Autodesk Inventor part; units mm, degrees
ref_plane "YZ Plane" through (0, 0, 0) normal (1, 0, 0) x (0, 1, 0)
ref_plane "XZ Plane" through (0, 0, 0) normal (0, 1, 0) x (-1, 0, 0)
ref_plane "XY Plane" through (0, 0, 0) normal (0, 0, 1) x (1, 0, 0)
sketch "Sketch1" plane through (0, 0, 0) normal (0, 1, 0) x (-1, 0, 0)
  point P0 (0, 0)
sketch "Sketch2" plane through (0, 0, 0) normal (0, 1, 0) x (-1, 0, 0)
  line L0 (-63.5, 112) -> (63.5, 112)
  line L1 (63.5, 112) -> (63.5, -112)
  line L2 (63.5, -112) -> (-63.5, -112)
  line L3 (-63.5, -112) -> (-63.5, 112)
  line L4 (-63.5, 112) -> (63.5, -112) construction
  line L5 (63.5, 112) -> (-63.5, -112) construction
  point P0 (0, 0)
  dimension "d0" = 127
  dimension "d1" = 224
extrude "Extrusion1" add sketch "Sketch2" along normal blind 76.2
sketch "Sketch3" plane through (0, 76.2, 0) normal (0, 1, 0) x (1, 0, 0)
  line L0 (59.69, 107.95) -> (-59.69, 107.95)
  line L1 (-59.69, 107.95) -> (-59.69, -107.95)
  line L2 (-59.69, -107.95) -> (59.69, -107.95)
  line L3 (59.69, -107.95) -> (59.69, 107.95)
  line L4 (59.69, 107.95) -> (-59.69, -107.95) construction
  line L5 (-59.69, 107.95) -> (59.69, -107.95) construction
  point P0 (0, 0)
  dimension "d4" = 119.38
  dimension "d5" = 215.9
extrude "Extrusion2" cut sketch "Sketch3" against normal blind 73.66
sketch "Sketch4" plane through (-59.69, 76.2, -107.95) normal (0, 0, 1) x (1, 0, 0)
  line L0 (119.38, 0) -> (119.38, -73.66)
  line L1 (119.38, 0) -> (0, 0)
  line L2 (0, 0) -> (0, -5.08)
  line L3 (0, -5.08) -> (119.38, -5.08)
  line L4 (119.38, -5.08) -> (119.38, 0)
  point P0 (59.69, -76.2)
  dimension "d8" = 5.08
  dimension "d11" = 119.38
extrude "Extrusion3" add sketch "Sketch4" along normal blind 38.1
sketch "Sketch5" plane through (59.69, 76.2, 107.95) normal (0, 0, -1) x (-1, 0, 0)
  line L0 (0, 0) -> (119.38, 0)
  line L1 (119.38, 0) -> (119.38, -5.08)
  line L2 (119.38, -5.08) -> (0, -5.08)
  line L3 (0, -5.08) -> (0, 0)
  point P0 (59.69, -76.2)
  dimension "d12" = 5.08
extrude "Extrusion4" add sketch "Sketch5" along normal blind 38.1
sketch "Sketch7" plane through (63.5, 0, 112) normal (1, 0, 0) x (0, 0, -1)
  line L0 (224, 0) -> (0, 0)
  line L1 (224, 0) -> (224, 76.2)
  line L2 (0, 76.2) -> (224, 76.2)
  line L3 (0, 0) -> (0, 76.2)
  point P0 (112, 0)
extrude "Extrusion5" cut sketch "Sketch7" against normal blind 5.08
sketch "Sketch8" plane through (-59.69, 76.2, -69.85) normal (0, 0, 1) x (1, 0, 0)
  line L0 (0, -5.08) -> (118.11, -5.08)
  line L1 (118.11, 0) -> (0, 0)
  line L2 (118.11, -5.08) -> (92.71, -5.08)
  line L3 (92.71, -5.08) -> (92.71, 0)
  line L4 (92.71, 0) -> (118.11, 0)
  line L5 (118.11, 0) -> (118.11, -5.08)
  point P0 (59.69, -76.2)
  dimension "d17" = 25.4
extrude "Extrusion6" add sketch "Sketch8" along normal blind 139.7
sketch "Sketch9" plane through (58.42, 0, 112) normal (1, 0, 0) x (0, 0, -1)
  line L0 (219.95, 2.54) -> (219.95, 71.12)
  line L1 (219.95, 2.54) -> (4.05, 2.54)
  line L2 (4.05, 2.54) -> (4.05, 0)
  line L3 (4.05, 0) -> (219.95, 0)
  line L4 (219.95, 0) -> (219.95, 2.54)
  point P0 (112, 0)
extrude "Extrusion7" cut sketch "Sketch9" against normal blind 71.12
fillet "Fillet1" radius 3.175 1 edges at (58.42, 71.12, 0)
fillet "Fillet2" radius 3.175 1 edges at (-13.335, 71.12, -69.85)
fillet "Fillet3" radius 3.175 1 edges at (-13.335, 71.12, 69.85)
sketch "Sketch10" plane through (-63.5, 0, -112) normal (0, 0, -1) x (-1, 0, 0)
  circle A0 centre (-102.87, 19.05) radius 4
  point P0 (-63.5, 0)
  dimension "d27" = 8
hole "Hole1" at (39.37, 19.05, -112) direction (0, 0, 1) diameter 8 end through all
fillet "Fillet4" radius 3.175 1 edges at (33.02, 71.12, 0)
sketch "Sketch11" plane through (-63.5, 0, 112) normal (0, 0, 1) x (1, 0, 0)
  point P0 (63.5, 0)
  point P1 (60.96, 12.7)
hole "Hole2" at (-2.54, 12.7, 112) direction (0, 0, -1) diameter 8 end through all
properties part number "Bucket des 1" material "ABS Plastic"
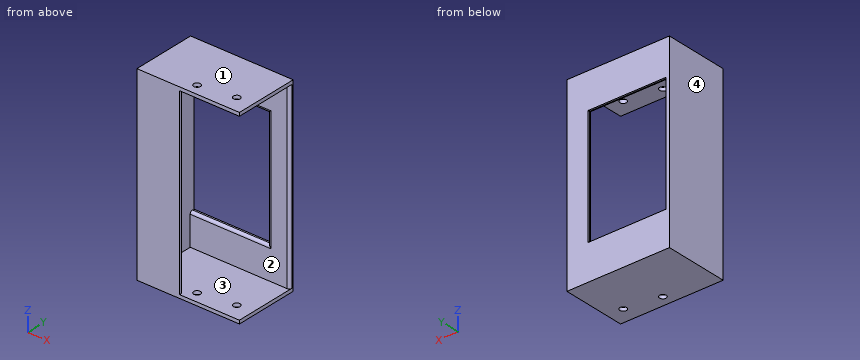
Model file for the job. Use its own axes, mm. Face numbers are marked on the shaded views. Round coordinates to 2 decimals unless told otherwise and drop trailing zeros. Loops run counter-clockwise (first coordinate to the right, second up) from the corner with the lowest first, then second, coordinate; pieces in that order, holes last. Notation, with made-up numbers: (20, -33.5) - (66, -33.5) arc R23 ccw to (66, -17.5) - close; hole circle Ø9 at (15.25, 27.25). An arc over 180 degrees is marked (long way). Write each question's results on one line, items separated by ' | '.
(1) Mould opens along Z. For the marked faces 1, 2, 3 and 4 say: released by +Z, released by -Z, zero draft, split by the parting line, or undercut.
Answer below:
face 1: released by +Z | face 2: undercut | face 3: undercut | face 4: zero draft
(2) Pin check, flat tips, straight feed: pin 1 (6.5 mm diameter, centred on x = 39.37, y = 19.05, fed in from +Z); pin 2 (5 mm diameter, centred on y = 28, z = -4, fed in from +X); pin 3 (4 mm diameter, centred on x = -21, z = -22.5, fed in from +Y); pin 4 (3 mm diameter, centred on y = 1.5, z = -1, fed in from +X). Stop position of each tip, or through.
Answer below:
pin 1: passes through | pin 2: stops at x = -59.69 | pin 3: stops at y = 2.54 | pin 4: stops at x = -12.7
(3) Wall check: L1, parallel to X at y = 19.05, z = -108.95; L2, parallel to Z at x = 7.5, y = 55.5; L3, parallel to Y at x = -2, z = -110. Give the ranges that are in metal, low to high.
Answer below:
L1: x = -63.5 to 35.37, 43.37 to 58.42 | L2: z = -112 to -107.95, 107.95 to 112 | L3: y = 0 to 8.74, 16.66 to 76.2
(4) Saw through at B-B, the plane z = -55. List the corners of the cut face in (x, y) (3 decimals), then the cut area to 3 significant figures.
Answer below:
outline: (-63.5, 0) - (-12.7, 0) - (-12.7, 2.54) - (-59.69, 2.54) - (-59.69, 76.2) - (-63.5, 76.2) - close; (33.02, 74.295) arc R3.175 ccw to (36.195, 71.12) - (55.245, 71.12) arc R3.175 ccw to (58.42, 74.295) - (58.42, 76.2) - (33.02, 76.2) - close | area: 534 mm^2
(5) Saw through at D-D, the plane x = -2.54. List the corners of the cut face in (y, z) (3 decimals).
Answer below:
outline: (0, -112) - (8.7, -112) - (8.7, -107.95) - (0, -107.95) - close; (0, 107.95) - (8.7, 107.95) - (8.7, 112) - (0, 112) - close; (16.7, -112) - (76.2, -112) - (76.2, -69.85) - (74.295, -69.85) arc R3.175 ccw to (71.12, -73.025) - (71.12, -107.95) - (16.7, -107.95) - close; (16.7, 107.95) - (71.12, 107.95) - (71.12, 73.025) arc R3.175 ccw to (74.295, 69.85) - (76.2, 69.85) - (76.2, 112) - (16.7, 112) - close
(6) Saw through at A-A, the plane x = 15. List the corners of the cut face in (y, z) (3 decimals), then the cut area to 4 significant figures.
Answer below:
outline: (0, -112) - (76.2, -112) - (76.2, -69.85) - (74.295, -69.85) arc R3.175 ccw to (71.12, -73.025) - (71.12, -107.95) - (0, -107.95) - close; (0, 107.95) - (71.12, 107.95) - (71.12, 73.025) arc R3.175 ccw to (74.295, 69.85) - (76.2, 69.85) - (76.2, 112) - (0, 112) - close | area: 1,000 mm^2
(7) Saw through at C-C, the plane y = 19.05. List the corners of the cut face in (x, z).
Answer below:
outline: (-63.5, -112) - (35.37, -112) - (35.37, -107.95) - (-59.69, -107.95) - (-59.69, 107.95) - (35.37, 107.95) - (35.37, 112) - (-63.5, 112) - close; (43.37, -112) - (58.42, -112) - (58.42, -107.95) - (43.37, -107.95) - close; (43.37, 107.95) - (58.42, 107.95) - (58.42, 112) - (43.37, 112) - close
